Model file for the job. Use its own axes, mm. A direction names the side the tool comes from. Give positions to 0.01 mm unless a question says otherwise; leave off trailing zeros. Write each loop counter-clockwise with the first axis right and the second up, starting at its lowest first coordinate (ties: lowest second). Pieces come first, ordered by that corner, then holes. Notation, with made-up numbers: (-40, 22) - (4, 22) arc R10 cw to (4, 32) - close; hole circle Ø1 at (64, 41). An arc over 180 degrees is marked (long way). Use CSV: the item, a comma, the result in double quotes.
Autodesk Inventor part; units mm, degrees
ref_plane "YZ Plane" through (0, 0, 0) normal (1, 0, 0) x (0, 1, 0)
ref_plane "XZ Plane" through (0, 0, 0) normal (0, 1, 0) x (-1, 0, 0)
ref_plane "XY Plane" through (0, 0, 0) normal (0, 0, 1) x (1, 0, 0)
sketch "Sketch1" plane through (0, 0, 0) normal (0, 0, 1) x (1, 0, 0)
  line L0 (11.5, -11.5) -> (-11.5, -11.5)
  line L1 (-11.5, -11.5) -> (-11.5, 11.5)
  line L2 (-11.5, 11.5) -> (11.5, 11.5)
  line L3 (11.5, 11.5) -> (11.5, -11.5)
  point P0 (0, 0)
  point P1 (0, 11.5)
  point P2 (-11.5, 0)
  dimension "d0" = 23
extrude "Extrusion1" add sketch "Sketch1" along normal blind 6
sketch "Sketch2" plane through (0, 0, 6) normal (0, 0, 1) x (1, 0, 0)
  circle A0 centre (0, 0) radius 4
  dimension "d3" = 8
extrude "Extrusion2" cut sketch "Sketch2" against normal blind 5
sketch "Sketch3" plane through (0, 0, 0) normal (0, 0, -1) x (-1, 0, 0)
  line L0 (11.5, 11.5) -> (11.5, -11.5)
  line L1 (11.5, -11.5) -> (4.5, -11.5)
  line L2 (4.5, -11.5) -> (4.5, -4.5)
  line L3 (4.5, -4.5) -> (11.5, -4.5)
  line L4 (11.5, -4.5) -> (11.5, -11.5)
  circle A0 centre (8, -8) radius 1.75
  point P0 (0, 0)
  dimension "d6" = 3.5
  dimension "d7" = 7
  dimension "d8" = 8
  dimension "d9" = 8
extrude "Extrusion3" add sketch "Sketch3" along normal blind 1.5
extrude "Extrusion4" add sketch "Sketch3" along normal blind 4.5 contours A0
pattern_circular "Circular Pattern1" count 4 over 360 about axis through (0, 0, -10) along (0, 0, 1) of "Extrusion3", "Extrusion4"
properties part number "AS5600 Testteil"
(1) Flat gauge pins, fed straight in: P1, Ø1.5, axis at x = 7.5, z = -2.5, coming from the +Y side; P2, Ø1, axis at x = 0, y = 2.5, coming from the -Z side. Where does each tip first touch, or does it go through?
Checked values:
P1,"stops at y = 9.75"
P2,"stops at z = 0"
(2) Saw through at A-A, the plane z = 3. List the corners of the cut face in (x, y).
Checked values:
outline,"(-11.5, -11.5) - (11.5, -11.5) - (11.5, 11.5) - (-11.5, 11.5) - close; hole circle Ø8 at (0, 0)"
(3) Wall check: probe 1 along Y at (x, z) = (0, 2.75); probe 2 along Y at (x, z) = (-5.5, -1); probe 3 along Z at (x, y) = (1.75, 1.25). Give the ranges that are in metal, low to high. Write a range as [from, to].
Checked values:
probe 1,"y = [-11.5, -4], [4, 11.5]"
probe 2,"y = [-11.5, -4.5], [4.5, 11.5]"
probe 3,"z = [0, 1]"
(4) Saw through at B-B, the plane y = 0. List the corners of the cut face in (x, z).
Checked values:
outline,"(-11.5, 0) - (11.5, 0) - (11.5, 6) - (4, 6) - (4, 1) - (-4, 1) - (-4, 6) - (-11.5, 6) - close"
(5) Saw through at D-D, the plane z = -3. List the corners of the cut face in (x, y).
Checked values:
outline,"circle Ø3.5 at (-8, -8); circle Ø3.5 at (-8, 8); circle Ø3.5 at (8, -8); circle Ø3.5 at (8, 8)"
(6) Pull direction Y, two halves, no side cores. Call faces 1 (the face through (8, -4.5, -1)), 2 (the face through (0, -11.5, 2)), 3 (the face through (-8, 8, -4.5)): released by +Y, released by -Y, zero draft, split by the parting line, or undercut.
Checked values:
face 1,"undercut"
face 2,"released by -Y"
face 3,"zero draft"
(7) 3-axis set-ups, long thin cutter, end or side, ignore diameter. For faces 4 (the face through (4.5, -8, -1)), 5 (the face through (0, 0, 1)), 6 (the face through (8.526, -9.669, -2.979)), 7 (the face through (11.5, 0, 2)), 8 (the face through (-8, -4.5, -1)): which of +Z, -Z, +X, -X, +Y, -Y reach the whole face in a straight line?
Checked values:
face 4,"-Z, +Y, -Y"
face 5,"+Z"
face 6,"-Z"
face 7,"+Z, -Z, +X, +Y, -Y"
face 8,"-Z, +X, -X"
(8) Saw through at C-C, the plane x = -8. List the corners of the cut face in (y, z), then the cut area to 3 significant figures.
Checked values:
outline,"(-11.5, -1.5) - (-9.75, -1.5) - (-9.75, -4.5) - (-6.25, -4.5) - (-6.25, -1.5) - (-4.5, -1.5) - (-4.5, 0) - (4.5, 0) - (4.5, -1.5) - (6.25, -1.5) - (6.25, -4.5) - (9.75, -4.5) - (9.75, -1.5) - (11.5, -1.5) - (11.5, 6) - (-11.5, 6) - close"
area,"180 mm^2"
